Here's how the part is built. I have some questions about the finished solid (model axes, mm). A direction names the side the tool comes from. Round coordinates to 2 decimals unless told otherwise and drop trailing zeros. Loops run counter-clockwise (first coordinate to the right, second up) from the corner with the lowest first, then second, coordinate; pieces in that order, holes last. Notation, with made-up numbers: (89, 65.5) - (106, 65.5) arc R27 cw to (106, 87.5) - close; hole circle Ø9 at (-18, 7.25). An arc over 180 degrees is marked (long way). Answer as a JSON object with one key per item and string values. Group by question number.
1) If we mould it in two halves opening along X, with no side actions, what happens to faces 1 (the face through (-0.12, -31.27, 1.48)), 2 (the face through (37.378, -5, 1)), 3 (the face through (-32.622, -5, 1))? For each: pulls with the +X half, pulls with the -X half, needs draft (parallel to the pull), parting line crosses it, or undercut.
2) I want a section at B-B, the plane x = 10. Please give me the cut outline in (y, z), then the cut area to 3 significant figures.
3) If I drill on line 1 along X through (y, z) = (21, 0.55); line 2 along X through (y, z) = (-16.5, 0.45); line 3 along X through (y, z) = (-31, 1.65), over which ranges is the centre line in solid material (lowest first)? Write a range as [from, to].
4) I want a section at C-C, the plane y = -31. Please give me the cut outline in (x, z).
5) Which directions (+Z, -Z, +X, -X, +Y, -Y) give clear straight access to the entire face, cutting with the end or side of a thin tool? Please do faces 4 (the face through (2, 30.336, 1)), 5 (the face through (2, 23.908, 1)).
6) I want a section at D-D, the plane y = 13. Please give me the cut outline in (x, z).
7) I want a section at A-A, the plane z = 1.4. Give the number of separate pieces and of enclosed holes in the cut face, then the cut area to 3 significant figures.
from build123d import *

# Parameters (mm, degrees)
ESBO_O1_W                = 70
ESBO_O1_H                = 70
RESSALTO_EXTRUS_O2_DEPTH = 3


with BuildPart() as part:
    # Esboço1 → Ressalto-extrusão2 (new body)
    with BuildSketch(Plane.XY):
        with Locations((2.378031716, -4.663986286)):
            Rectangle(ESBO_O1_W, ESBO_O1_H)
        with BuildLine():
            ThreePointArc((-26.193742937, -2.999482116), (-24.193742937, -2.163986286), (-22.193742937, -2.999482116))
            Line((-22.193742937, -2.999482116), (-22.193742937, -6.328490456))
            ThreePointArc((-22.193742937, -6.328490456), (-24.193742937, -7.163986286), (-26.193742937, -6.328490456))
            Line((-26.193742937, -6.328490456), (-26.193742937, -2.999482116))
        make_face(mode=Mode.SUBTRACT)
        with BuildLine():
            Line((4.042535886, -33.235760939), (0.713527546, -33.235760939))
            ThreePointArc((0.713527546, -33.235760939), (-0.121968284, -31.235760939), (0.713527546, -29.235760939))
            Line((0.713527546, -29.235760939), (4.042535886, -29.235760939))
            ThreePointArc((4.042535886, -29.235760939), (4.878031716, -31.235760939), (4.042535886, -33.235760939))
        make_face(mode=Mode.SUBTRACT)
        Polygon((0.256711372, -4.663986286), (-25.19913275, 20.791857837), (-23.077812407, 22.91317818), (2.378031716, -2.542665942), (27.833875839, 22.91317818), (29.955196182, 20.791857837), (4.499352059, -4.663986286), (29.955196182, -30.119830409), (27.833875839, -32.241150752), (2.378031716, -6.78530663), (-23.077812407, -32.241150752), (-25.19913275, -30.119830409), align=None, mode=Mode.SUBTRACT)
        with BuildLine():
            Line((26.949806369, -6.328490456), (26.949806369, -2.999482116))
            ThreePointArc((26.949806369, -2.999482116), (28.949806369, -2.163986286), (30.949806369, -2.999482116))
            Line((30.949806369, -2.999482116), (30.949806369, -6.328490456))
            ThreePointArc((30.949806369, -6.328490456), (28.949806369, -7.163986286), (26.949806369, -6.328490456))
        make_face(mode=Mode.SUBTRACT)
        with BuildLine():
            ThreePointArc((0.713527546, 19.907788367), (-0.121968284, 21.907788367), (0.713527546, 23.907788367))
            Line((0.713527546, 23.907788367), (4.042535886, 23.907788367))
            ThreePointArc((4.042535886, 23.907788367), (4.878031716, 21.907788367), (4.042535886, 19.907788367))
            Line((4.042535886, 19.907788367), (0.713527546, 19.907788367))
        make_face(mode=Mode.SUBTRACT)
    extrude(amount=RESSALTO_EXTRUS_O2_DEPTH)


solid = part.part
Outcome:
{
 "1": {"face 1": "undercut", "face 2": "pulls with the +X half", "face 3": "pulls with the -X half"},
 "2": {"outline": "(-39.66, 0) - (-14.41, 0) - (-14.41, 3) - (-39.66, 3) - close; (-10.16, 0) - (0.84, 0) - (0.84, 3) - (-10.16, 3) - close; (5.08, 0) - (30.34, 0) - (30.34, 3) - (5.08, 3) - close", "area": "185 mm^2"},
 "3": {"line 1": "[-32.62, -24.99], [-21.16, 0.03], [4.73, 25.92], [29.75, 37.38]", "line 2": "[-32.62, -11.58], [-7.34, 12.09], [16.34, 37.38]", "line 3": "[-32.62, -24.32], [-21.84, -0.11], [4.87, 26.59], [29.08, 37.38]"},
 "4": {"outline": "(-32.62, 0) - (-24.32, 0) - (-24.32, 3) - (-32.62, 3) - close; (-21.84, 0) - (-0.11, 0) - (-0.11, 3) - (-21.84, 3) - close; (4.87, 0) - (26.59, 0) - (26.59, 3) - (4.87, 3) - close; (29.08, 0) - (37.38, 0) - (37.38, 3) - (29.08, 3) - close"},
 "5": {"face 4": "+Z, -Z, +X, -X, +Y", "face 5": "+Z, -Z"},
 "6": {"outline": "(-32.62, 0) - (-17.41, 0) - (-17.41, 3) - (-32.62, 3) - close; (-13.16, 0) - (17.92, 0) - (17.92, 3) - (-13.16, 3) - close; (22.16, 0) - (37.38, 0) - (37.38, 3) - (22.16, 3) - close"},
 "7": {"separate pieces": "1", "enclosed holes": "5", "area": "4,390 mm^2"}
}
